from build123d import *

# Parameters (mm, degrees)
F0_R     = 6.985
F1_DEPTH = 2.032
F2_R     = 5.715
F3_DEPTH = 2.54
F4_R     = 6.985
F5_DEPTH = 2.032
F6_R     = 2.54
F7_DEPTH = 12.7


with BuildPart() as f1:
    # F0 (on Front) → F1 (new body)
    with BuildSketch(Plane.XZ):
        Circle(F0_R)
    extrude(amount=F1_DEPTH)

    # F2 (on face) → F3 (join)
    with BuildSketch(Plane.XZ.offset(2.032)):
        Circle(F2_R)
    extrude(amount=F3_DEPTH)

    # F4 (on face) → F5 (join)
    with BuildSketch(Plane.XZ.offset(4.572)):
        Circle(F4_R)
    extrude(amount=F5_DEPTH)

    # F6 (on face) → F7 (cut, symmetric)
    with BuildSketch(Plane.XZ.offset(6.604)):
        Circle(F6_R)
    extrude(amount=F7_DEPTH, both=True, mode=Mode.SUBTRACT)


solid = f1.part
The listing builds one solid part. Answer for the finished solid, in the listing's coordinates (mm). A direction names the side the tool comes from. Coordinates: 2 decimals unless noted, no trailing zeros. Loops run counter-clockwise (first coordinate to the right, second up) from the corner with the lowest first, then second, coordinate; pieces in that order, holes last.
1) Find the intervals of material crossed by L1, parallel to Z at x = 0, y = -1.25 (3 decimals); L2, parallel to Z at x = 0, y = -3.75 (3 decimals); L3, parallel to Y at x = 2.25, z = 5.75, in increasing order.
2) Find section C-C on y = -1. Write down the section's boundary in (x, z) (3 decimals), then the cut area to 3 significant figures.
3) A tool of negligible diameter and unlimited length cuts with its end or side. For faces 4 (the face through (-6, -4.572, 0)), 5 (the face through (3, -6.604, 0)), from which of +Z, -Z, +X, -X, +Y, -Y can it reach the whole face along a straight path? Write none if from no direction.
4) Find section D-D on x = -5.25. Write down the section's boundary in (y, z).
5) Find section A-A on z = 0. Write down the section's boundary in (x, y) (3 decimals), then the cut area to 3 significant figures.
6) Determine the mould class of faces 1 (the face through (-0.33, -3.35, 2.52)), 2 (the face through (-0.909, -5.574, 6.926)), 3 (the face through (-6, -2.032, 0)) for opening direction X: pulls with the +X half, pulls with the -X half, needs draft (parallel to the pull), parting line crosses it, or undercut.
7) Find section B-B on x = 0. Write down the section's boundary in (y, z) (3 decimals).
8) Flat-ended cylindrical pins translate along their axes: pin 1 Ø1.5 at (x, y) = (3, -3) entering from -Z; pin 2 Ø3 at (x, z) = (0, 0) entering from +Y (1 decimal). Find the tip coordinate at first contact, or state that the pin passes through.
Values:
1. L1: z = -6.985 to -2.54, 2.54 to 6.985
1. L2: z = -5.715 to -2.54, 2.54 to 5.715
1. L3: y = -6.6 to -4.57, -2.03 to 0
2. outline: circle Ø13.97 at (0, 0); hole circle Ø5.08 at (0, 0)
2. area: 133 mm2
3. face 4: none
3. face 5: +Z, -Z, +X, -X, -Y
4. outline: (-6.6, -4.61) - (-4.57, -4.61) - (-4.57, -2.26) - (-2.03, -2.26) - (-2.03, -4.61) - (0, -4.61) - (0, 4.61) - (-2.03, 4.61) - (-2.03, 2.26) - (-4.57, 2.26) - (-4.57, 4.61) - (-6.6, 4.61) - close
5. outline: (-6.985, -6.604) - (-2.54, -6.604) - (-2.54, 0) - (-6.985, 0) - (-6.985, -2.032) - (-5.715, -2.032) - (-5.715, -4.572) - (-6.985, -4.572) - close; (2.54, -6.604) - (6.985, -6.604) - (6.985, -4.572) - (5.715, -4.572) - (5.715, -2.032) - (6.985, -2.032) - (6.985, 0) - (2.54, 0) - close
5. area: 52.3 mm2
6. face 1: undercut
6. face 2: parting line crosses it
6. face 3: needs draft
7. outline: (-6.604, -6.985) - (-4.572, -6.985) - (-4.572, -5.715) - (-2.032, -5.715) - (-2.032, -6.985) - (0, -6.985) - (0, -2.54) - (-6.604, -2.54) - close; (-6.604, 2.54) - (0, 2.54) - (0, 6.985) - (-2.032, 6.985) - (-2.032, 5.715) - (-4.572, 5.715) - (-4.572, 6.985) - (-6.604, 6.985) - close
8. pin 1: stops at z = -5.25
8. pin 2: passes through
